```python
from build123d import *

# Parameters (mm, degrees)
F0_R     = 32.6923124251
F1_DEPTH = 14.6508645266
F2_W     = 224.4729697704
F2_H     = 29.9537181854
F3_DEPTH = 10.0321955979
F3_TAPER = -3
F4_R     = 40.1130157543
F5_DEPTH = 18.4948313981
F7_D     = 63.5
F7_DEPTH = 50.8
F7_TIP   = 19.0773246541
F8_DEPTH = 11.372352019


with BuildPart() as f1:
    # F0 (on Front) → F1 (new body)
    with BuildSketch(Plane.XZ):
        Circle(F0_R)
    extrude(amount=F1_DEPTH)

    # F2 (on Front) → F3 (join)
    with BuildSketch(Plane.XZ):
        Rectangle(F2_W, F2_H)
    extrude(amount=F3_DEPTH, taper=F3_TAPER)

    # F4 (on Front) → F5 (join)
    with BuildSketch(Plane.XZ):
        Circle(F4_R)
    extrude(amount=F5_DEPTH)

    # F7
    with Locations(Plane(origin=(0, 0, 0), x_dir=(1, 0, 0), z_dir=(0, 1, 0))):
        with Locations((0, 0)):
            Hole(F7_D / 2, depth=F7_DEPTH)
            with Locations((0, 0, -(F7_DEPTH + F7_TIP / 2))):  # 118° drill point
                Cone(0, F7_D / 2, F7_TIP, mode=Mode.SUBTRACT)

    # F0 (on Front) → F8 (join)
    with BuildSketch(Plane.XZ):
        Circle(F0_R)
    extrude(amount=F8_DEPTH)


solid = f1.part
```
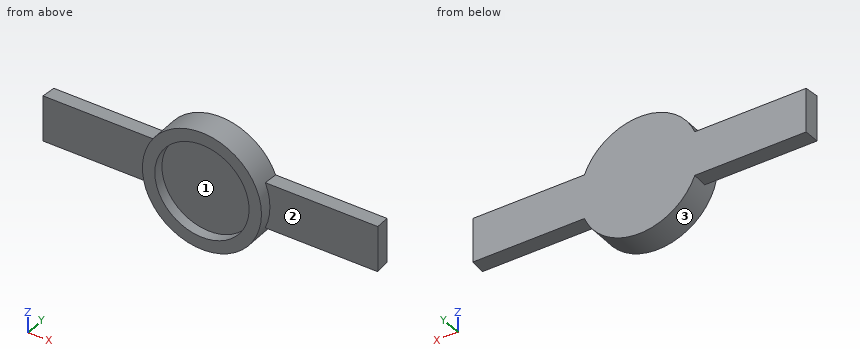
CAD build for the part. Positions are in the model's coordinates, mm. Face numbers are marked on the shaded views. Round coordinates to 2 decimals unless told otherwise and drop trailing zeros. Write each loop counter-clockwise with the first axis right and the second up, starting at its lowest first coordinate (ties: lowest second). Pieces come first, ordered by that corner, then holes.
Item 1: Drop flat-ended pins along their axis: pin 1 Ø25 at (x, z) = (84.5, -4.5) entering from -Y; pin 2 Ø6 at (x, y) = (-12.5, -14.5) entering from +Z; pin 3 Ø5 at (y, z) = (-7.5, -31.5) entering from -X. Give the stop position or say it passes through.
Filled in:
pin 1: stops at y = -10.03
pin 2: stops at z = 38.97
pin 3: stops at x = -27.71
Item 2: Mould opens along X. For the marked faces 1, 2 and 3 say: released by +X, released by -X, zero draft, split by the parting line, or undercut.
Filled in:
face 1: undercut
face 2: zero draft
face 3: split by the parting line
Item 3: Drill centre lines: L1, parallel to Z at x = 0, y = -14.75; L2, parallel to Z at x = 58.5, y = -10; L3, parallel to Y at x = -45.5, z = -7. Where is each one in solid material? Low to high.
Filled in:
L1: z = -40.11 to -31.75, 31.75 to 40.11
L2: z = -15.5 to 15.5
L3: y = -10.03 to 0
Item 4: Band-saw the part on B-B on z = -28. Write the cut outline in (x, y), then the cut area to 3 significant figures.
Filled in:
outline: (-28.72, -18.49) - (-14.97, -18.49) - (-14.97, -11.37) - (14.97, -11.37) - (14.97, -18.49) - (28.72, -18.49) - (28.72, 0) - (-28.72, 0) - close
area: 849 mm2
Item 5: Band-saw the part on A-A on x = 0. Write the cut outline in (y, z).
Filled in:
outline: (-18.49, -40.11) - (0, -40.11) - (0, 40.11) - (-18.49, 40.11) - (-18.49, 31.75) - (-11.37, 31.75) - (-11.37, -31.75) - (-18.49, -31.75) - close
